Here's how the part is built. I have some questions about the finished solid (model axes, mm). Give positions to 0.01 mm unless a question says otherwise; leave off trailing zeros. Loops run counter-clockwise (first coordinate to the right, second up) from the corner with the lowest first, then second, coordinate; pieces in that order, holes last. Notation, with made-up numbers: (75, 12.25) - (123, 12.25) arc R20 ccw to (123, 23.25) - close; hole circle Ø11 at (26.5, -15). An arc over 180 degrees is marked (long way). Use a Markdown table: item, result.
from build123d import *

# Parameters (mm, degrees)
F0_W     = 170
F0_H     = 258
F0_R     = 6.25
F0_R_2   = 17.5
F1_DEPTH = 15
F2_SIZE2 = 5
F2_SIZE  = 5


with BuildPart() as f1:
    # F0 (on Front) → F1 (new body)
    with BuildSketch(Plane.XZ):
        with Locations((-25, 0)):
            Rectangle(F0_W, F0_H)
        with Locations((-41.5, -41.5)):
            Circle(F0_R, mode=Mode.SUBTRACT)
        with Locations((41.5, -41.5)):
            Circle(F0_R, mode=Mode.SUBTRACT)
        with Locations((-32.5, 0)):
            Circle(F0_R, mode=Mode.SUBTRACT)
        with Locations((-41.5, 41.5)):
            Circle(F0_R, mode=Mode.SUBTRACT)
        Circle(F0_R_2, mode=Mode.SUBTRACT)
        with Locations((32.5, 0)):
            Circle(F0_R, mode=Mode.SUBTRACT)
        with Locations((41.5, 41.5)):
            Circle(F0_R, mode=Mode.SUBTRACT)
    extrude(amount=F1_DEPTH)

    # F2
    f2_edges = [f1.edges().sort_by_distance(p)[0] for p in [
        (-47.75, -15, 41.5),
        (35.25, -15, 41.5),
        (-47.75, -15, -41.5),
        (35.25, -15, -41.5),
        (60, -15, 0),
    ]]
    chamfer(f2_edges, length=F2_SIZE, length2=F2_SIZE2)


solid = f1.part
(1) Suppose I cut it at D-D on x = -41.5. Write out the boundary of the cut face in (y, z), plus the area to 4 significant figures.
A:
| item | result |
|---|---|
| outline | (-15, -129) - (0, -129) - (0, -47.75) - (-10, -47.75) - (-15, -52.75) - close; (-15, -30.25) - (-10, -35.25) - (0, -35.25) - (0, 35.25) - (-10, 35.25) - (-15, 30.25) - close; (-15, 52.75) - (-10, 47.75) - (0, 47.75) - (0, 129) - (-15, 129) - close |
| area | 3,445 mm2 |
(2) Will these pins go through, and if not, where does the flat tip stop? pin 1 (10 mm diameter, centred on x = -41.5, z = 41.5, fed in from +Y); pin 2 (12 mm diameter, centred on x = 16.5, z = 55.5, fed in from +Y).
A:
| item | result |
|---|---|
| pin 1 | through |
| pin 2 | y = 0 |
(3) Suppose I cut it at C-C on z = 0. Write out the boundary of the cut face in (x, y).
A:
| item | result |
|---|---|
| outline | (-110, -15) - (-38.75, -15) - (-38.75, 0) - (-110, 0) - close; (-26.25, -15) - (-17.5, -15) - (-17.5, 0) - (-26.25, 0) - close; (17.5, -15) - (26.25, -15) - (26.25, 0) - (17.5, 0) - close; (38.75, -15) - (55, -15) - (60, -10) - (60, 0) - (38.75, 0) - close |
(4) Suppose I cut it at B-B on x = 0. Write out the boundary of the cut face in (y, z), plus the area to 4 significant figures.
A:
| item | result |
|---|---|
| outline | (-15, -129) - (0, -129) - (0, -17.5) - (-15, -17.5) - close; (-15, 17.5) - (0, 17.5) - (0, 129) - (-15, 129) - close |
| area | 3,345 mm2 |
(5) Suppose I cut it at A-A on z = 41.5. Write out the boundary of the cut face in (x, y).
A:
| item | result |
|---|---|
| outline | (-110, -15) - (-52.75, -15) - (-47.75, -10) - (-47.75, 0) - (-110, 0) - close; (-35.25, -10) - (-30.25, -15) - (30.25, -15) - (35.25, -10) - (35.25, 0) - (-35.25, 0) - close; (47.75, -10) - (52.75, -15) - (55, -15) - (60, -10) - (60, 0) - (47.75, 0) - close |
(6) If I drill on line 1 (Z direction, x = 41.5, y = -7.5); line 2 (Z direction, x = 0, y = -6.5); line 3 (Z direction, x = 43.5, y = -4.75), over which ranges is the centre line in solid material (lowest first)?
A:
| item | result |
|---|---|
| line 1 | -129 to -47.75, -35.25 to 35.25, 47.75 to 129 |
| line 2 | -129 to -17.5, 17.5 to 129 |
| line 3 | -129 to -47.42, -35.58 to 35.58, 47.42 to 129 |
